Source: three-view drawing plus pictorial views. Frame: mm from the lowest corner of the part. Coordinates: 2 decimals unless noted, no trailing zeros. Write each loop counter-clockwise with the first axis right and the second up, starting at its lowest first coordinate (ties: lowest second). Pieces come first, ordered by that corner, then holes. Notation, with made-up numbers: M 65.25,35.5 L 96.25,35.5 A33 ccw 96.25,69.5 Z; hole C -39,-0.75 d9. An arc over 180 degrees is marked long. Write item = value, one per line. Start each with the question number.
Item 1: Section B-B on z = 6.25. Output: boundary loops of the cut face in (x, y), plus the area to 3 significant figures.
Item 2: Section A-A on y = 315. Output: boundary loops of the cut face in (x, z), plus the area to 3 significant figures.
Item 3: Section C-C on x = 40. Output: boundary loops of the cut face in (y, z).
Item 4: Pull-direction query (Y, two-part tool) for the marked faces 1, 2, 3 and 4; classes: +Y half, -Y half, draft (parallel to the pull), parting line (faces both ways), or undercut.
Item 5: Section D-D on x = 26.5. Output: boundary loops of the cut face in (y, z).
Item 6: Ray query, L1, parallel to Y at x = 40, z = 6; L2, parallel to Y at x = 35, z = 1.75 (3 decimals); L3, parallel to Y at x = 29, z = 1.25. Return the intervals inside material, ascending. Write a range as [from, to].
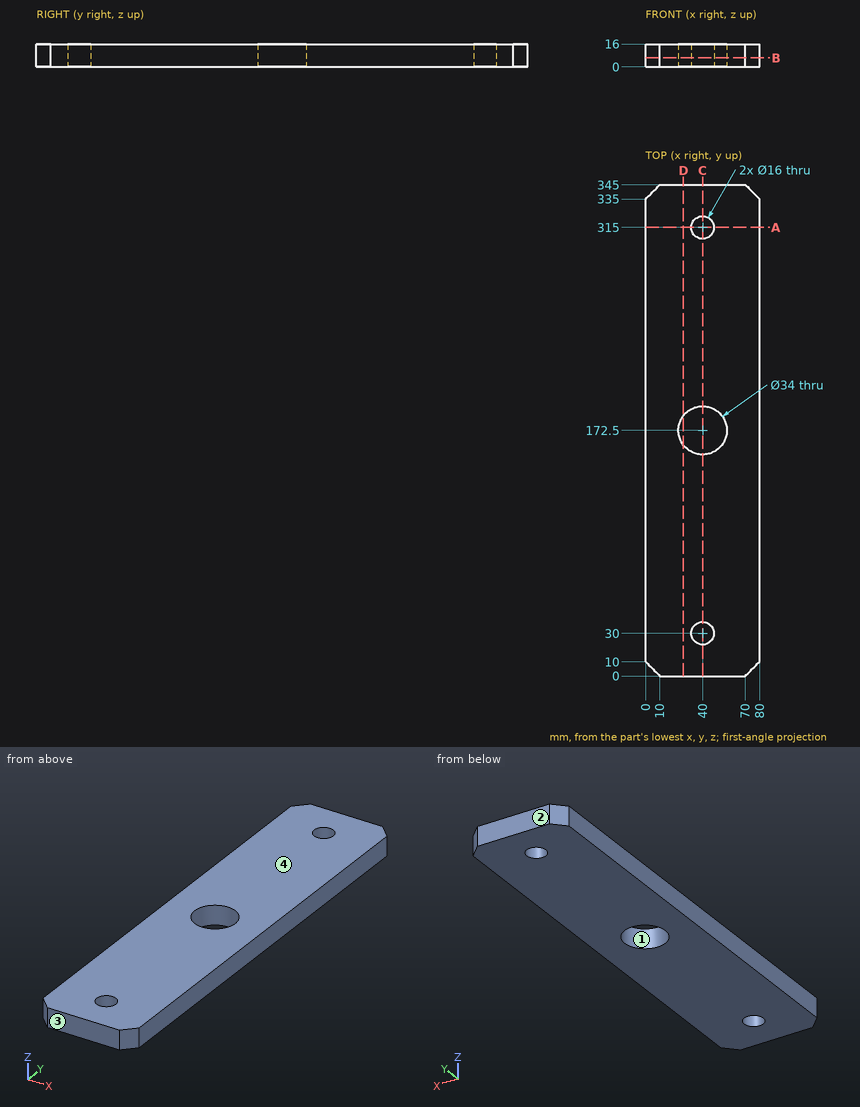
Responses:
q1.outline = M 0,10 L 10,0 L 70,0 L 80,10 L 80,335 L 70,345 L 10,345 L 0,335 Z; hole C 40,172.5 d34; hole C 40,30 d16; hole C 40,315 d16
q1.area = 26,100 mm²
q2.outline = M 0,0 L 32,0 L 32,16 L 0,16 Z; M 48,0 L 80,0 L 80,16 L 48,16 Z
q2.area = 1,020 mm²
q3.outline = M 0,0 L 22,0 L 22,16 L 0,16 Z; M 38,0 L 155.5,0 L 155.5,16 L 38,16 Z; M 189.5,0 L 307,0 L 307,16 L 189.5,16 Z; M 323,0 L 345,0 L 345,16 L 323,16 Z
q4.face_1 = undercut
q4.face_2 = +Y half
q4.face_3 = -Y half
q4.face_4 = draft
q5.outline = M 0,0 L 162.17,0 L 162.17,16 L 0,16 Z; M 182.83,0 L 345,0 L 345,16 L 182.83,16 Z
q6.L1 = [0, 22], [38, 155.5], [189.5, 307], [323, 345]
q6.L2 = [0, 23.755], [36.245, 156.252], [188.748, 308.755], [321.245, 345]
q6.L3 = [0, 159.54], [185.46, 345]
